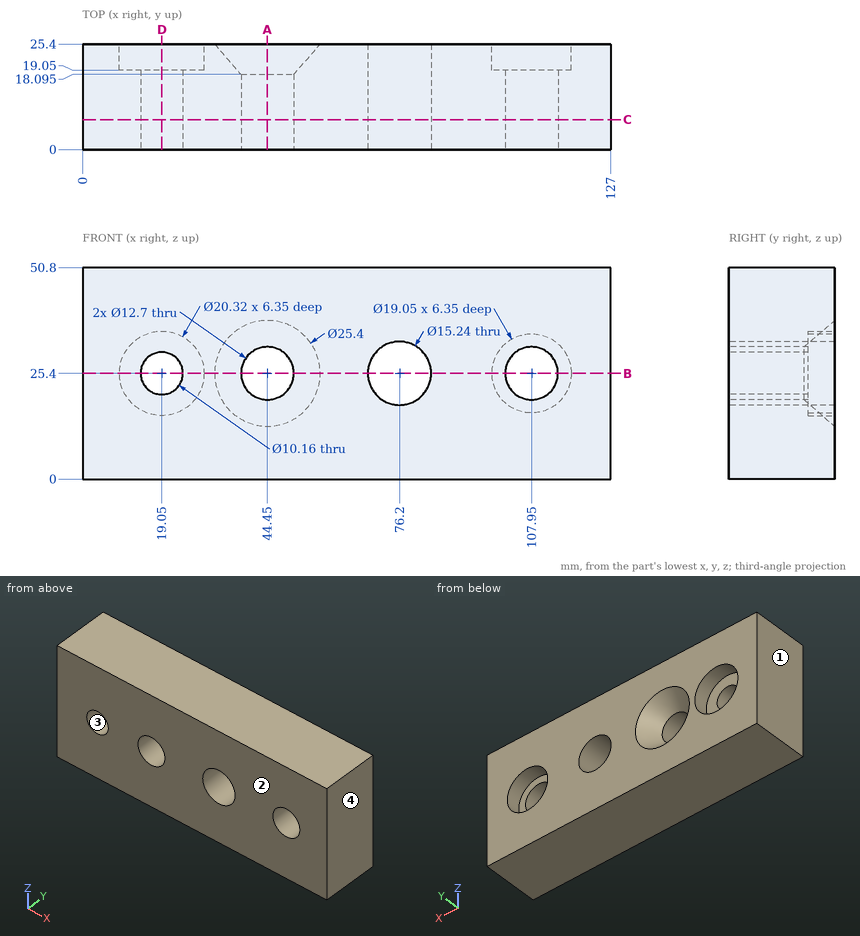
Study the drawing (mm; zero at the part's minimum x, y, z) and answer. Coordinates: 2 decimals unless noted, no trailing zeros. Loops run counter-clockwise (first coordinate to the right, second up) from the corner with the lowest first, then second, coordinate; pieces in that order, holes last. Notation, with made-up numbers: (-14.75, 28.25) -> (22.25, 28.25) arc R15 ccw to (22.25, 42.25) -> close; hole circle Ø8 at (-37, 80). An arc over 180 degrees is marked (long way). Answer in a Markdown table with one row per item. Add a question column.
1. The part is cut by section D-D, the plane x = 19.05. Write down the section's boundary in (y, z).
2. The part is cut by section A-A, the plane x = 44.45. Write down the section's boundary in (y, z) (3 decimals).
3. The part is cut by section B-B, the plane z = 25.4. Count the separate pieces of the cut face and the enclosed holes in it, then the cut area to 3 significant figures.
4. Consider line 1 (Z direction, x = 107.95, y = 11.25); line 2 (Z direction, x = 107.95, y = 22.5) (3 decimals); line 3 (X direction, y = 21, z = 31) (1 decimal). Determine where each line is inside the solid, lowest interval first. Write a range as [from, to].
5. Determine the mould class of the marked faces 1, 2, 3 and 4 for opening direction X: +X half, -X half, draft (parallel to the pull), parting line (faces both ways), or undercut.
6. The part is cut by section C-C, the plane y = 7.25. Write down the section's boundary in (x, z), then the cut area to 3 significant figures.
Answer below:
| question | item | result |
|---|---|---|
| 1 | outline | (0, 0) -> (25.4, 0) -> (25.4, 15.24) -> (19.05, 15.24) -> (19.05, 20.32) -> (0, 20.32) -> close; (0, 30.48) -> (19.05, 30.48) -> (19.05, 35.56) -> (25.4, 35.56) -> (25.4, 50.8) -> (0, 50.8) -> close |
| 2 | outline | (0, 0) -> (25.4, 0) -> (25.4, 12.7) -> (18.095, 19.05) -> (0, 19.05) -> close; (0, 31.75) -> (18.095, 31.75) -> (25.4, 38.1) -> (25.4, 50.8) -> (0, 50.8) -> close |
| 3 | separate pieces | 5 |
| 3 | enclosed holes | 0 |
| 3 | area | 1,780 mm2 |
| 4 | line 1 | [0, 19.05], [31.75, 50.8] |
| 4 | line 2 | [0, 15.875], [34.925, 50.8] |
| 4 | line 3 | [0, 10.6], [27.5, 37.6], [51.3, 71], [81.4, 100.2], [115.7, 127] |
| 5 | face 1 | -X half |
| 5 | face 2 | draft |
| 5 | face 3 | undercut |
| 5 | face 4 | +X half |
| 6 | outline | (0, 0) -> (127, 0) -> (127, 50.8) -> (0, 50.8) -> close; hole circle Ø10.16 at (19.05, 25.4); hole circle Ø12.7 at (44.45, 25.4); hole circle Ø15.24 at (76.2, 25.4); hole circle Ø12.7 at (107.95, 25.4) |
| 6 | area | 5,930 mm2 |
